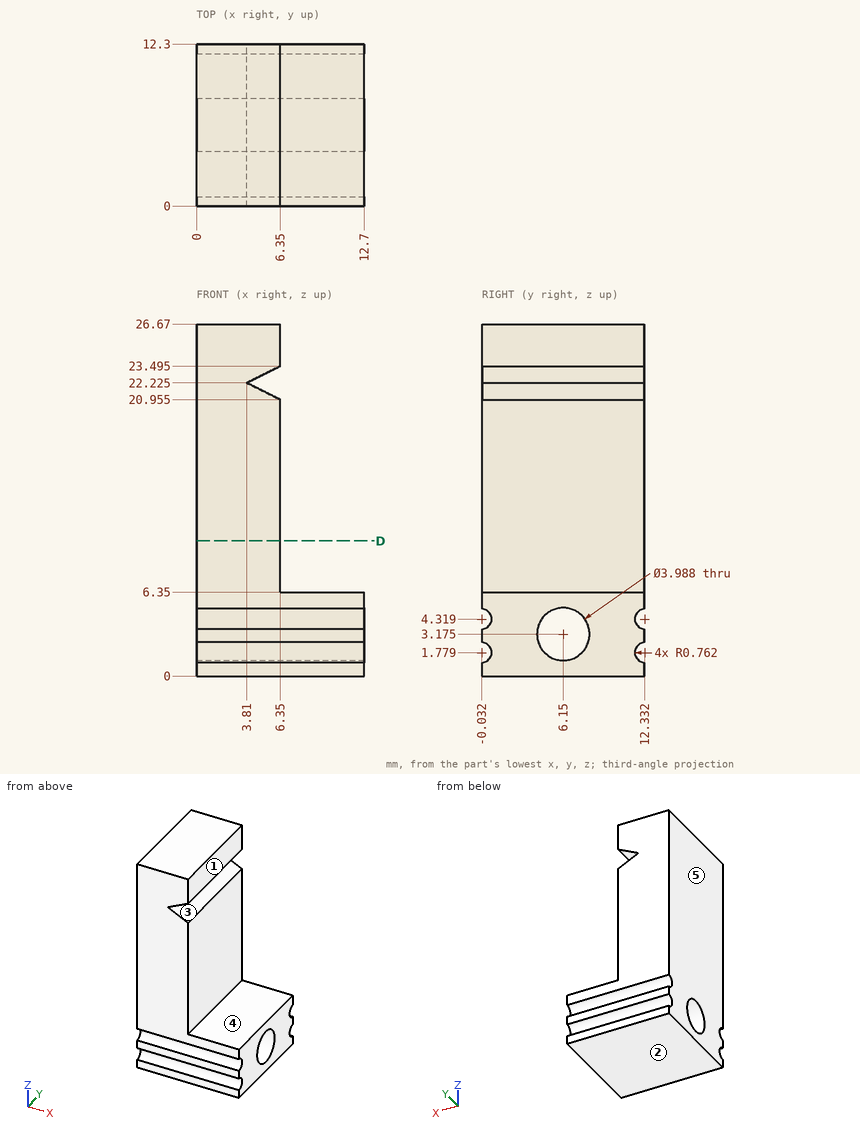
The figure shows three views and two pictorial views of one solid part (mm, origin at its lowest corner). Answer the questions. A direction names the side the tool comes from. Give positions to 0.01 mm unless a question says otherwise; leave off trailing zeros. Write each loop counter-clockwise with the first axis right and the second up, starting at its lowest first coordinate (ties: lowest second). Pieces come first, ordered by that corner, then holes. Notation, with made-up numbers: (67, 51) - (113, 51) arc R9 cw to (113, 55) - close; hole circle Ø6 at (-26, 68). An arc over 180 degrees is marked (long way). Use one line per item in the form item = value. Start each with the question number.
1) Consider line 1 along Z through (x, y) = (7.5, 6.15); line 2 along Z through (x, y) = (3, 6.15); line 3 along Z through (x, y) = (5.25, 6.15) (1 decimal). Determine where each line is inside the solid, lowest interval first. Write a range as from..to.
2) Flat-ended cylindrical pins translate along their axes: pin 1 Ø1 at (y, z) = (5.5, 25) entering from +X; pin 2 Ø6 at (x, y) = (10, 4.5) entering from +Z. Find the tip coordinate at first contact, or state that the pin passes through.
3) The mould has two halves that part along Z. Classify the marked faces 3, 4 and 5: pulls with the +Z half, pulls with the -Z half, needs draft (parallel to the pull), parting line crosses it, or undercut.
4) A tool of negligible diameter and unlimited length cuts with its end or side. For the marked faces 1 and 2, from which of +Z, -Z, +X, -X, +Y, -Y can it reach the whole face along a straight path? Write none if from no direction.
5) Find section D-D on z = 10.25. Determine the outline of the cut face in (x, y).
Geometry results:
q1.line_1 = 0..1.18, 5.17..6.35
q1.line_2 = 0..1.18, 5.17..26.67
q1.line_3 = 0..1.2, 5.2..21.5, 22.9..26.7
q2.pin_1 = 6.35
q2.pin_2 = 6.35
q3.face_3 = undercut
q3.face_4 = pulls with the +Z half
q3.face_5 = needs draft
q4.face_1 = +Z, +X, +Y, -Y
q4.face_2 = -Z, +X, -X, +Y, -Y
q5.outline = (0, 0) - (6.35, 0) - (6.35, 12.3) - (0, 12.3) - close
